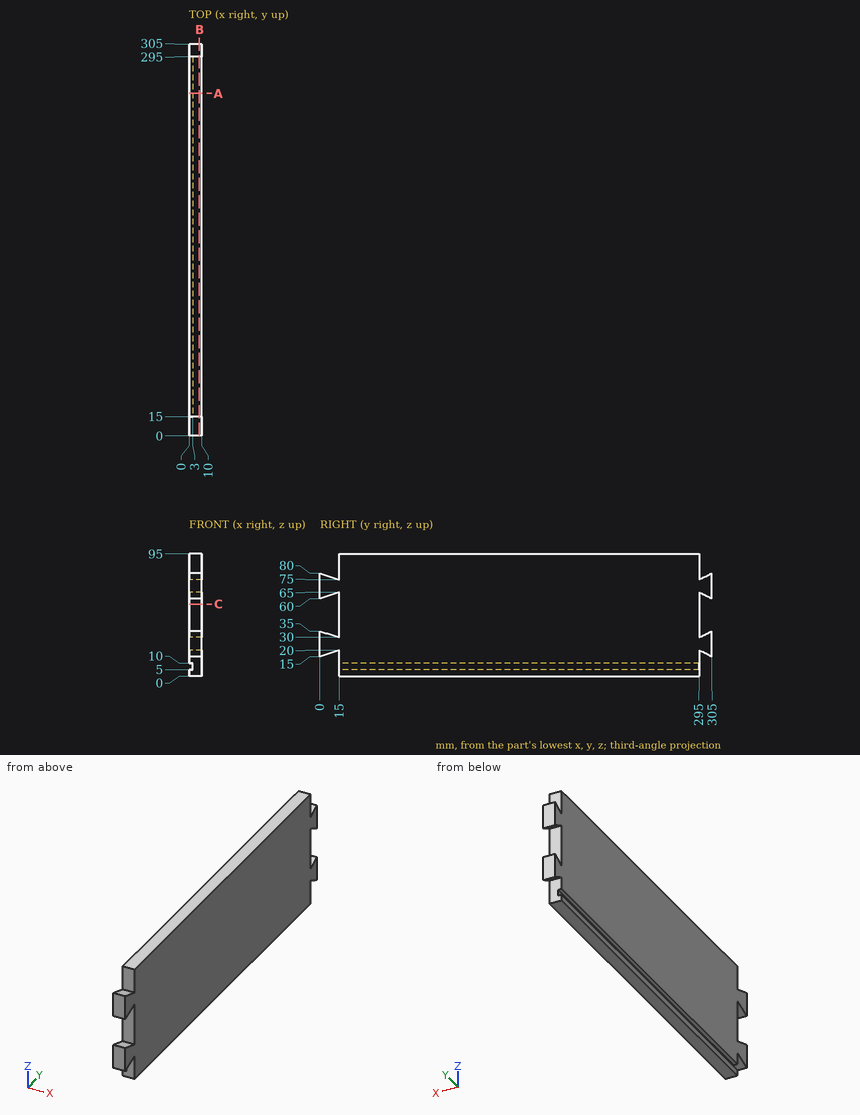
Geometry: see drawing. Coordinates: mm, zero at the bounding-box minimum. Coordinates: 2 decimals unless noted, no trailing zeros. Order: outer loops, then holes, each group sorted by start corner. A loop starts at its lowest first (then second) coordinate and runs counter-clockwise, first axis right, second up. Notation, with made-up numbers: M 67,10 L 95,10 A14 ccw 95,21 Z; hole C 69,64 d5. An arc over 180 degrees is marked long. Answer in a Markdown table with one row per item. Add a question column.
Q1. Line query: L1, parallel to Y at x = 2.25, z = 42. Output: solid intervals per line, ascending.
Q2. Section query A-A on y = 266.5. Return the cut outline in (x, z).
Q3. Section query B-B on x = 8. Return the cut outline in (y, z), and give its area (4 significant figures).
Q4. Contact query for flat-ended pins moving along their axis: P1, Ø0.9, axis at x = 2, y = 128, coming from the -Z side; P2, Ø5, axis at x = 5.5, z = 83, coming from the -Y side; P3, Ø3, axis at x = 3, z = 43.5, coming from the +Y side. Output: stop coordinate, or through.
Q5. Section query C-C on z = 56. Return the cut outline in (x, y), and give its area (3 significant figures).
Completed:
| question | item | result |
|---|---|---|
| 1 | L1 | y = 15 to 295 |
| 2 | outline | M 0,0 L 10,0 L 10,95 L 0,95 L 0,10 L 3,10 L 3,5 L 0,5 Z |
| 3 | outline | M 0,15 L 15,20 L 15,0 L 295,0 L 295,20 L 305,15 L 305,35 L 295,30 L 295,65 L 305,60 L 305,80 L 295,75 L 295,95 L 15,95 L 15,75 L 0,80 L 0,60 L 15,65 L 15,30 L 0,35 Z |
| 3 | area | 27,350 mm2 |
| 4 | P1 | stops at z = 0 |
| 4 | P2 | stops at y = 15 |
| 4 | P3 | stops at y = 295 |
| 5 | outline | M 0,15 L 10,15 L 10,295 L 0,295 Z |
| 5 | area | 2,800 mm2 |
